Autodesk Inventor part; units mm, degrees
ref_plane "YZ Plane" through (0, 0, 0) normal (1, 0, 0) x (0, 1, 0)
ref_plane "XZ Plane" through (0, 0, 0) normal (0, 1, 0) x (-1, 0, 0)
ref_plane "XY Plane" through (0, 0, 0) normal (0, 0, 1) x (1, 0, 0)
sketch "Sketch2" plane through (0, 0, 0) normal (0, 0, 1) x (1, 0, 0)
  line L0 (0, 0) -> (-9.9, 0)
  line L1 (-4.95, 0) -> (-4.95, 2.5)
  line L2 (-4.95, 0) -> (-2.45, 0) construction
  circle A0 centre (-4.95, 5) radius 2.5
  line L3 (-4.95, 7.5) -> (32.05, 7.5) construction
  line L4 (0, 0) -> (-9.9, 0)
  line L5 (0, 0) -> (-9.9, 0)
  line L6 (-4.95, 7.5) -> (66.05, 7.5) construction
  line L7 (-4.95, 7.5) -> (70.05, 7.5) construction
  line L8 (0, 0) -> (-9.9, 0)
  line L9 (-9.9, 0) -> (-9.9, 82.5)
  line L10 (0, 82.5) -> (0, 0)
  line L11 (0, 82.5) -> (0, 85.5)
  line L12 (0, 85.5) -> (-9.9, 85.5)
  line L13 (-9.9, 85.5) -> (-9.9, 82.5)
  dimension "d35" = 5
  dimension "d33" = 2.5
  dimension "d34" = 90
  dimension "d48" = 9.9
  dimension "d49" = 9.9
  dimension "d50" = 3
extrude "Extrusion6" add sketch "Sketch2" along normal blind 5
properties part number "Cube_Holder_SB_V1_(71mm)"
Work out the finished part from the listing and answer in its coordinate system (mm). Give positions to 0.01 mm unless a question says otherwise; leave off trailing zeros. Loops run counter-clockwise (first coordinate to the right, second up) from the corner with the lowest first, then second, coordinate; pieces in that order, holes last. Notation, with made-up numbers: (-23.75, -1) -> (17.25, -1) arc R27 cw to (17.25, 20) -> close; hole circle Ø11 at (13, 61.25). An arc over 180 degrees is marked (long way). Put each result on its own line as item: value. Start each with the question number.
Item 1: The part is cut by section C-C (z = 1.6). Give the vertices of the cut face in (x, y), then the cut area to 3 significant figures.
Item 2: Find the intervals of material crossed by L1, parallel to X at y = 5, z = 3.75; L2, parallel to Y at x = -4.95, z = 1.85; L3, parallel to Y at x = -6.75, z = 3.8, in increasing order. Write a range as [from, to].
Item 3: The part is cut by section B-B (x = -4.95). Give the vertices of the cut face in (y, z), then the cut area to 4 significant figures.
Item 4: The part is cut by section A-A (y = 5). Give the vertices of the cut face in (x, z).
Answers below:
1. outline: (-9.9, 0) -> (0, 0) -> (0, 85.5) -> (-9.9, 85.5) -> close; hole circle Ø5 at (-4.95, 5)
1. area: 827 mm2
2. L1: [-9.9, -7.45], [-2.45, 0]
2. L2: [0, 2.5], [7.5, 85.5]
2. L3: [0, 3.27], [6.73, 85.5]
3. outline: (0, 0) -> (2.5, 0) -> (2.5, 5) -> (0, 5) -> close; (7.5, 0) -> (85.5, 0) -> (85.5, 5) -> (7.5, 5) -> close
3. area: 402.5 mm2
4. outline: (-9.9, 0) -> (-7.45, 0) -> (-7.45, 5) -> (-9.9, 5) -> close; (-2.45, 0) -> (0, 0) -> (0, 5) -> (-2.45, 5) -> close
